from build123d import *

# Parameters (mm, degrees)
SALIENTE_EXTRUIR2_DEPTH    = 10
CROQUIS3_R                 = 9.947805623
SALIENTE_EXTRUIR3_DEPTH    = 1
CORTAR_EXTRUIR1_DEPTH      = 68.948509917
CORTAR_EXTRUIR1_DEPTH_BACK = 68.948509917
CROQUIS4_R                 = 5.8
SALIENTE_EXTRUIR4_DEPTH    = 9
CORTAR_EXTRUIR2_DEPTH      = 83.807004535
CORTAR_EXTRUIR2_DEPTH_BACK = 83.807004535
REDONDEO3_START            = -10.0000001
REDONDEO3_DEPTH            = 1.0000001
REDONDEO3_START_2          = 9
REDONDEO3_2_DEPTH          = 1
REDONDEO3_START_3          = -9
REDONDEO3_3_DEPTH          = 18
REDONDEO3_START_4          = -29.193321254
REDONDEO3_4_DEPTH          = 58.386642508
REDONDEO4_R                = 4


with BuildPart() as part:
    # Croquis2 → Saliente-Extruir2 (new, symmetric)
    with BuildSketch(Plane.XY):
        with BuildLine():
            Line((-49, 0), (-49, 46))
            Line((-49, 46), (49, 46))
            Line((49, 46), (49, 0))
            Line((49, 0), (28.8, 0))
            ThreePointArc((28.8, 0), (0, 28.8), (-28.8, 0))
            Line((-28.8, 0), (-49, 0))
        make_face()
    extrude(amount=SALIENTE_EXTRUIR2_DEPTH, both=True)

    # Croquis3 → Saliente-Extruir3 (add)
    with BuildSketch(Plane(origin=(0, 46, 0), x_dir=(1, 0, 0), z_dir=(0, 1, 0))):
        with Locations(Location((-39.052194377, 0.052194377, 0), (0, 0, 90))):
            Circle(CROQUIS3_R)
        with Locations(Location((39.052194377, 0.052194377, 0), (0, 0, 90))):
            Circle(CROQUIS3_R)
    extrude(amount=SALIENTE_EXTRUIR3_DEPTH)

    # Croquis4 → Cortar-Extruir1 (cut, two sides: drawn at the far end of the back side and taken through both)
    with BuildSketch(Plane(origin=(0, 46, 0), x_dir=(1, 0, 0), z_dir=(0, 1, 0)).offset(-CORTAR_EXTRUIR1_DEPTH_BACK)):
        with Locations(Location((-39.052194377, 0.052194377, 0), (0, 0, 270))):
            Circle(CROQUIS4_R)
        with Locations(Location((39.052194377, 0.052194377, 0), (0, 0, 270))):
            Circle(CROQUIS4_R)
    extrude(amount=CORTAR_EXTRUIR1_DEPTH + CORTAR_EXTRUIR1_DEPTH_BACK, mode=Mode.SUBTRACT)

    # Croquis5 → Saliente-Extruir4 (add, symmetric)
    with BuildSketch(Plane.XY):
        with BuildLine():
            Line((-28.5, 46), (28.5, 46))
            ThreePointArc((28.5, 46), (0, 66), (-28.5, 46))
        make_face()
    extrude(amount=SALIENTE_EXTRUIR4_DEPTH, both=True)

    # Croquis6 → Cortar-Extruir2 (cut, two sides: drawn at the far end of the back side and taken through both)
    with BuildSketch(Plane(origin=(0, 0, 0), x_dir=(0, 0, -1), z_dir=(1, 0, 0)).offset(-CORTAR_EXTRUIR2_DEPTH_BACK)):
        with BuildLine():
            Line((-9, 66), (-9, 54))
            add(Edge.make_bspline(
                [(-9, 54), (-6.728088744, 61.714285714), (-5, 66)],
                knots=[0, 0, 0, 0.174230423, 0.174230423, 0.174230423], degree=2, weights=[1, 1.104611797, 1.172770478]))
            Line((-5, 66), (-9, 66))
        make_face()
        with BuildLine():
            add(Edge.make_bspline(
                [(5, 66), (6.728088744, 61.714285714), (9, 54)],
                knots=[0.825769577, 0.825769577, 0.825769577, 1, 1, 1], degree=2, weights=[1.172770478, 1.104611797, 1]))
            Line((9, 54), (9, 66))
            Line((9, 66), (5, 66))
        make_face()
    extrude(amount=CORTAR_EXTRUIR2_DEPTH + CORTAR_EXTRUIR2_DEPTH_BACK, mode=Mode.SUBTRACT)

    # Redondeo3: read off the stored shape, not the designer's step
    # Redondeo3 outline → Redondeo3 (add)
    with BuildSketch(Plane.XY.offset(REDONDEO3_START)):
        with BuildLine():
            Line((-29.193321154, 46), (29.193321154, 46))
            ThreePointArc((29.193321154, 46), (28.62814416, 46.175030325), (28.260813391, 46.63885007))
            ThreePointArc((28.260813391, 46.63885007), (0, 66), (-28.260813391, 46.63885007))
            ThreePointArc((-28.260813391, 46.63885007), (-28.62814416, 46.175030325), (-29.193321154, 46))
        make_face()
    extrude(amount=REDONDEO3_DEPTH)

    # Redondeo3 2 outline → Redondeo3 2 (add)
    with BuildSketch(Plane.XY.offset(REDONDEO3_START_2)):
        with BuildLine():
            Line((-29.193321154, 46), (29.193321154, 46))
            ThreePointArc((29.193321154, 46), (28.62814416, 46.175030325), (28.260813391, 46.63885007))
            ThreePointArc((28.260813391, 46.63885007), (0, 66), (-28.260813391, 46.63885007))
            ThreePointArc((-28.260813391, 46.63885007), (-28.62814416, 46.175030325), (-29.193321154, 46))
        make_face()
    extrude(amount=REDONDEO3_2_DEPTH)

    # Redondeo3 3 outline → Redondeo3 3 (add)
    with BuildSketch(Plane.XY.offset(REDONDEO3_START_3)):
        with BuildLine():
            ThreePointArc((-28.5, 46), (-28.382204223, 46.320098033), (-28.260813391, 46.63885007))
            ThreePointArc((-28.260813391, 46.63885007), (-28.62814416, 46.175030325), (-29.193321154, 46))
            Line((-29.193321154, 46), (-28.5, 46))
        make_face()
        with BuildLine():
            ThreePointArc((29.193321154, 46), (28.62814416, 46.175030325), (28.260813391, 46.63885007))
            ThreePointArc((28.260813391, 46.63885007), (28.382204223, 46.320098033), (28.5, 46))
            Line((28.5, 46), (29.193321154, 46))
        make_face()
    extrude(amount=REDONDEO3_3_DEPTH)

    # Redondeo3 4 outline → Redondeo3 4 (cut)
    with BuildSketch(Plane.YZ.offset(REDONDEO3_START_4)):
        with BuildLine():
            Line((47, 9), (67, 9))
            Line((67, 9), (67, 10))
            Line((67, 10), (46, 10))
            ThreePointArc((46, 10), (46.292893219, 9.292893219), (47, 9))
        make_face()
        with BuildLine():
            Line((67, -10), (67, -9))
            Line((67, -9), (47, -9))
            ThreePointArc((47, -9), (46.292893219, -9.292893219), (46, -10))
            Line((46, -10), (67, -10))
        make_face()
    extrude(amount=REDONDEO3_4_DEPTH, mode=Mode.SUBTRACT)

    # Redondeo4
    redondeo4_edges = [part.edges().sort_by_distance(p)[0] for p in [
        (49, 23, 10),
        (-49, 23, 10),
        (-49, 23, -10),
        (49, 23, -10),
    ]]
    fillet(redondeo4_edges, radius=REDONDEO4_R)


solid = part.part
The listing builds one solid part. Answer for the finished solid, in the listing's coordinates (mm). A direction names the side the tool comes from. Coordinates: 2 decimals unless noted, no trailing zeros. Loops run counter-clockwise (first coordinate to the right, second up) from the corner with the lowest first, then second, coordinate; pieces in that order, holes last.
1) Find section B-B on x = 31.5. Write down the section's boundary in (y, z), then the cut area to 3 significant figures.
2) Determine the mould class of faces 1 (the face through (1, 34, 10)), 2 (the face through (47.797, 22.678, 8.859)), 3 (the face through (0.633, 28.793, 0.14)) for opening direction X: pulls with the +X half, pulls with the -X half, needs draft (parallel to the pull), parting line crosses it, or undercut.
3) Find the intervals of material crossed by L1, parallel to X at y = 40, z = -1; L2, parallel to Y at x = -31, z = 9.25; L3, parallel to X at y = 4, z = -4, in increasing order.
4) Find section A-A on y = 39. Write down the section's boundary in (x, z).
5) Flat-ended cylindrical pins translate along their axes: pin 1 Ø8 at (x, z) = (35.5, 3) entering from +Y; pin 2 Ø4 at (y, z) = (20.5, 7) entering from +X; pin 3 Ø1 at (x, z) = (-10.5, 7.5) entering from -Y; pin 4 Ø5.5 at (x, y) = (-4.5, 51.5) entering from +Z. Find the tip coordinate at first contact, or state that the pin passes through.
6) A tool of negligible diameter and unlimited length cuts with its end or side. For faces 4 (the face through (-47, 46, -8)), 5 (the face through (29.19, 46.49, 1.24)), 6 (the face through (36.1, 46, 9.8)), 7 (the face through (47, 46, -8)), 8 (the face through (0, 50, 9)), from which of +Z, -Z, +X, -X, +Y, -Y can it reach the whole face along a straight path? Write none if from no direction.
7) Find section C-C on y = 50. Write down the section's boundary in (x, z).
Values:
1. outline: (0, -10) - (46, -10) - (46, -6.53) - (47, -6.53) - (47, 6.42) - (46, 6.42) - (46, 10) - (0, 10) - close
1. area: 933 mm2
2. face 1: needs draft
2. face 2: pulls with the +X half
2. face 3: undercut
3. L1: x = -49 to -44.77, -33.33 to 33.33, 44.77 to 49
3. L2: y = 0 to 46
3. L3: x = -49 to -43.3, -34.8 to -28.52, 28.52 to 34.8, 43.3 to 49
4. outline: (-49, -6) arc R4 ccw to (-45, -10) - (45, -10) arc R4 ccw to (49, -6) - (49, 6) arc R4 ccw to (45, 10) - (-45, 10) arc R4 ccw to (-49, 6) - close; hole circle Ø11.6 at (-39.05, -0.05); hole circle Ø11.6 at (39.05, -0.05)
5. pin 1: stops at y = 47
5. pin 2: stops at x = 49
5. pin 3: stops at y = 26.62
5. pin 4: stops at z = 9
6. face 4: -Z, -X, +Y
6. face 5: +Y
6. face 6: +Z, +Y
6. face 7: -Z, +X, +Y
6. face 8: +Z, +X, -X, +Y
7. outline: (-26.72, -9) - (26.72, -9) - (26.72, 9) - (-26.72, 9) - close
